Read the model definition and answer for the solid it produces. Units are mm, in the model's axes. Coordinates: 2 decimals unless noted, no trailing zeros. Order: outer loops, then holes, each group sorted by start corner. A loop starts at its lowest first (then second) coordinate and runs counter-clockwise, first axis right, second up. Notation, with made-up numbers: (1.5, 56.5) -> (22.5, 56.5) arc R6 ccw to (22.5, 65.5) -> close; hole circle Ø2 at (19, 4). An arc over 180 degrees is marked (long way). Answer as a JSON object with one key per item and string values. Group by question number.
1) Consider L1, parallel to Y at x = -84, z = 1.65; L2, parallel to Y at x = -152, z = 4.25; L3, parallel to X at y = 238, z = 2.35. Determine where each line is inside the solid, lowest interval first.
2) Section B-B on x = -83 is taken. Determine the outline of the cut face in (y, z).
3) Section A-A on y = 238.5 is taken. Determine the outline of the cut face in (x, z), and give its area (3 significant figures).
4) Section C-C on y = 31 is taken. Determine the outline of the cut face in (x, z).
5) Given pin 1 (1.5 mm diameter, centred on x = -56.5, z = 1.5, fed in from -Y); pin 2 (3 mm diameter, centred on x = -52, z = 2, fed in from +Y), each flat-ended and moving along its own axis, determine where each tip first touches the part or whether it passes through.
6) Section D-D on z = 3.7 is taken. Count the separate pieces of the cut face and the enclosed holes in it, and give its area (3 significant figures).
from build123d import *

# Parameters (mm, degrees)
BASE_DEPTH                = 5
ESQUISSE3_R               = 2
ESQUISSE3_W               = 65
ESQUISSE3_H               = 30
ENL_V_MAT_EXTRU_1_DEPTH   = 6
CONG_1_R                  = 3
PER_AGE_POUR_BILLES_REACH = 7
ESQUISSE6_R               = 2
ESQUISSE6_R_2             = 11
PER_AGE_POUR_PROFIL_REACH = 7
ESQUISSE8_R               = 3
ESQUISSE10_R              = 2
ENL_V_MAT_EXTRU_3_DEPTH   = 6
ESQUISSE13_R              = 2
ENL_V_MAT_EXTRU_4_DEPTH   = 10


with BuildPart() as part:
    # Esquisse1 → Base (new body)
    with BuildSketch(Plane.XY):
        Polygon((0, 0), (-175, 0), (-199.748737342, 24.748737342), (-199.748737342, 284.748737342), (-175, 309.497474683), (0, 309.497474683), (24.748737342, 284.748737342), (24.748737342, 24.748737342), align=None)
    extrude(amount=BASE_DEPTH)

    # Esquisse3 → Enlèv. mat.-Extru.1 (cut, through all)
    with BuildSketch(Plane(origin=(0, 0, 0), x_dir=(-1, 0, 0), z_dir=(0, 0, -1))):
        with Locations((52.5, 45)):
            Circle(ESQUISSE3_R)
        with Locations((122.5, 45)):
            Circle(ESQUISSE3_R)
        with Locations((122.5, 264.497474683)):
            Circle(ESQUISSE3_R)
        with Locations((52.5, 264.497474683)):
            Circle(ESQUISSE3_R)
        Polygon((129.5, 0), (129.5, 20), (105.5, 20), (105.5, 45.5), (69.5, 45.5), (69.5, 20), (45.5, 20), (45.5, 0), align=None)
        Polygon((45.5, 309.497474683), (129.5, 309.497474683), (129.5, 289.497474683), (105.5, 289.497474683), (105.5, 263.997474683), (69.5, 263.997474683), (69.5, 289.497474683), (45.5, 289.497474683), align=None)
        with Locations((87.5, 239.497474683)):
            Rectangle(ESQUISSE3_W, ESQUISSE3_H)
        with Locations((87.5, 70)):
            Rectangle(ESQUISSE3_W, ESQUISSE3_H)
    extrude(amount=-ENL_V_MAT_EXTRU_1_DEPTH, mode=Mode.SUBTRACT)

    # Congé1
    cong_1_edges = [part.edges().sort_by_distance(p)[0] for p in [
        (0, 0, 2.5),
        (-175, 0, 2.5),
        (-199.748737342, 24.748737342, 2.5),
        (-199.748737342, 284.748737342, 2.5),
        (-175, 309.497474683, 2.5),
        (0, 309.497474683, 2.5),
        (24.748737342, 284.748737342, 2.5),
        (24.748737342, 24.748737342, 2.5),
        (-45.5, 289.497474683, 2.5),
        (-45.5, 309.497474683, 2.5),
        (-129.5, 309.497474683, 2.5),
        (-129.5, 289.497474683, 2.5),
        (-105.5, 289.497474683, 2.5),
        (-105.5, 263.997474683, 2.5),
        (-69.5, 263.997474683, 2.5),
        (-69.5, 289.497474683, 2.5),
        (-129.5, 0, 2.5),
        (-45.5, 0, 2.5),
        (-45.5, 20, 2.5),
        (-69.5, 20, 2.5),
        (-69.5, 45.5, 2.5),
        (-105.5, 45.5, 2.5),
        (-105.5, 20, 2.5),
        (-129.5, 20, 2.5),
    ]]
    fillet(cong_1_edges, radius=CONG_1_R)

    # Esquisse6 → Perçage pour billes (cut, up to next)
    with BuildSketch(Plane.XY.offset(5), mode=Mode.PRIVATE) as per_age_pour_billes_sk1:
        with Locations((-1.784271247, 16)):
            Circle(ESQUISSE6_R)
    per_age_pour_billes_tool1 = extrude(per_age_pour_billes_sk1.sketch, amount=-PER_AGE_POUR_BILLES_REACH, mode=Mode.PRIVATE) & part.part
    add(per_age_pour_billes_tool1.solids().sort_by_distance((-1.784271, 16, 5))[0], mode=Mode.SUBTRACT)
    # Esquisse6 → Perçage pour billes (cut, up to next)
    with BuildSketch(Plane.XY.offset(5), mode=Mode.PRIVATE) as per_age_pour_billes_sk2:
        with Locations((-1.784271247, 46)):
            Circle(ESQUISSE6_R)
    per_age_pour_billes_tool2 = extrude(per_age_pour_billes_sk2.sketch, amount=-PER_AGE_POUR_BILLES_REACH, mode=Mode.PRIVATE) & part.part
    add(per_age_pour_billes_tool2.solids().sort_by_distance((-1.784271, 46, 5))[0], mode=Mode.SUBTRACT)
    # Esquisse6 → Perçage pour billes (cut, up to next)
    with BuildSketch(Plane.XY.offset(5), mode=Mode.PRIVATE) as per_age_pour_billes_sk3:
        with Locations((-1.784271247, 263.497474683)):
            Circle(ESQUISSE6_R)
    per_age_pour_billes_tool3 = extrude(per_age_pour_billes_sk3.sketch, amount=-PER_AGE_POUR_BILLES_REACH, mode=Mode.PRIVATE) & part.part
    add(per_age_pour_billes_tool3.solids().sort_by_distance((-1.784271, 263.497475, 5))[0], mode=Mode.SUBTRACT)
    # Esquisse6 → Perçage pour billes (cut, up to next)
    with BuildSketch(Plane.XY.offset(5), mode=Mode.PRIVATE) as per_age_pour_billes_sk4:
        with Locations((-1.784271247, 293.497474683)):
            Circle(ESQUISSE6_R)
    per_age_pour_billes_tool4 = extrude(per_age_pour_billes_sk4.sketch, amount=-PER_AGE_POUR_BILLES_REACH, mode=Mode.PRIVATE) & part.part
    add(per_age_pour_billes_tool4.solids().sort_by_distance((-1.784271, 293.497475, 5))[0], mode=Mode.SUBTRACT)
    # Esquisse6 → Perçage pour billes (cut, up to next)
    with BuildSketch(Plane.XY.offset(5), mode=Mode.PRIVATE) as per_age_pour_billes_sk5:
        with Locations((-1.784271247, 278.497474683)):
            Circle(ESQUISSE6_R_2)
    per_age_pour_billes_tool5 = extrude(per_age_pour_billes_sk5.sketch, amount=-PER_AGE_POUR_BILLES_REACH, mode=Mode.PRIVATE) & part.part
    add(per_age_pour_billes_tool5.solids().sort_by_distance((-1.784271, 278.497475, 5))[0], mode=Mode.SUBTRACT)
    # Esquisse6 → Perçage pour billes (cut, up to next)
    with BuildSketch(Plane.XY.offset(5), mode=Mode.PRIVATE) as per_age_pour_billes_sk6:
        with Locations((-1.784271247, 31)):
            Circle(ESQUISSE6_R_2)
    per_age_pour_billes_tool6 = extrude(per_age_pour_billes_sk6.sketch, amount=-PER_AGE_POUR_BILLES_REACH, mode=Mode.PRIVATE) & part.part
    add(per_age_pour_billes_tool6.solids().sort_by_distance((-1.784271, 31, 5))[0], mode=Mode.SUBTRACT)
    # Esquisse6 → Perçage pour billes (cut, up to next)
    with BuildSketch(Plane.XY.offset(5), mode=Mode.PRIVATE) as per_age_pour_billes_sk7:
        with Locations((-173.215728753, 16)):
            Circle(ESQUISSE6_R)
    per_age_pour_billes_tool7 = extrude(per_age_pour_billes_sk7.sketch, amount=-PER_AGE_POUR_BILLES_REACH, mode=Mode.PRIVATE) & part.part
    add(per_age_pour_billes_tool7.solids().sort_by_distance((-173.215729, 16, 5))[0], mode=Mode.SUBTRACT)
    # Esquisse6 → Perçage pour billes (cut, up to next)
    with BuildSketch(Plane.XY.offset(5), mode=Mode.PRIVATE) as per_age_pour_billes_sk8:
        with Locations((-173.215728753, 46)):
            Circle(ESQUISSE6_R)
    per_age_pour_billes_tool8 = extrude(per_age_pour_billes_sk8.sketch, amount=-PER_AGE_POUR_BILLES_REACH, mode=Mode.PRIVATE) & part.part
    add(per_age_pour_billes_tool8.solids().sort_by_distance((-173.215729, 46, 5))[0], mode=Mode.SUBTRACT)
    # Esquisse6 → Perçage pour billes (cut, up to next)
    with BuildSketch(Plane.XY.offset(5), mode=Mode.PRIVATE) as per_age_pour_billes_sk9:
        with Locations((-173.215728753, 31)):
            Circle(ESQUISSE6_R_2)
    per_age_pour_billes_tool9 = extrude(per_age_pour_billes_sk9.sketch, amount=-PER_AGE_POUR_BILLES_REACH, mode=Mode.PRIVATE) & part.part
    add(per_age_pour_billes_tool9.solids().sort_by_distance((-173.215729, 31, 5))[0], mode=Mode.SUBTRACT)
    # Esquisse6 → Perçage pour billes (cut, up to next)
    with BuildSketch(Plane.XY.offset(5), mode=Mode.PRIVATE) as per_age_pour_billes_sk10:
        with Locations((-173.215728753, 263.497474683)):
            Circle(ESQUISSE6_R)
    per_age_pour_billes_tool10 = extrude(per_age_pour_billes_sk10.sketch, amount=-PER_AGE_POUR_BILLES_REACH, mode=Mode.PRIVATE) & part.part
    add(per_age_pour_billes_tool10.solids().sort_by_distance((-173.215729, 263.497475, 5))[0], mode=Mode.SUBTRACT)
    # Esquisse6 → Perçage pour billes (cut, up to next)
    with BuildSketch(Plane.XY.offset(5), mode=Mode.PRIVATE) as per_age_pour_billes_sk11:
        with Locations((-173.215728753, 293.497474683)):
            Circle(ESQUISSE6_R)
    per_age_pour_billes_tool11 = extrude(per_age_pour_billes_sk11.sketch, amount=-PER_AGE_POUR_BILLES_REACH, mode=Mode.PRIVATE) & part.part
    add(per_age_pour_billes_tool11.solids().sort_by_distance((-173.215729, 293.497475, 5))[0], mode=Mode.SUBTRACT)
    # Esquisse6 → Perçage pour billes (cut, up to next)
    with BuildSketch(Plane.XY.offset(5), mode=Mode.PRIVATE) as per_age_pour_billes_sk12:
        with Locations((-173.215728753, 278.497474683)):
            Circle(ESQUISSE6_R_2)
    per_age_pour_billes_tool12 = extrude(per_age_pour_billes_sk12.sketch, amount=-PER_AGE_POUR_BILLES_REACH, mode=Mode.PRIVATE) & part.part
    add(per_age_pour_billes_tool12.solids().sort_by_distance((-173.215729, 278.497475, 5))[0], mode=Mode.SUBTRACT)

    # Esquisse8 → Perçage pour profilé (cut, up to next)
    with BuildSketch(Plane.XY.offset(5), mode=Mode.PRIVATE) as per_age_pour_profil_sk1:
        with Locations((-152.5, 23)):
            Circle(ESQUISSE8_R)
    per_age_pour_profil_tool1 = extrude(per_age_pour_profil_sk1.sketch, amount=-PER_AGE_POUR_PROFIL_REACH, mode=Mode.PRIVATE) & part.part
    add(per_age_pour_profil_tool1.solids().sort_by_distance((-152.5, 23, 5))[0], mode=Mode.SUBTRACT)
    # Esquisse8 → Perçage pour profilé (cut, up to next)
    with BuildSketch(Plane.XY.offset(5), mode=Mode.PRIVATE) as per_age_pour_profil_sk2:
        with Locations((-152.5, 286.497474683)):
            Circle(ESQUISSE8_R)
    per_age_pour_profil_tool2 = extrude(per_age_pour_profil_sk2.sketch, amount=-PER_AGE_POUR_PROFIL_REACH, mode=Mode.PRIVATE) & part.part
    add(per_age_pour_profil_tool2.solids().sort_by_distance((-152.5, 286.497475, 5))[0], mode=Mode.SUBTRACT)
    # Esquisse8 → Perçage pour profilé (cut, up to next)
    with BuildSketch(Plane.XY.offset(5), mode=Mode.PRIVATE) as per_age_pour_profil_sk3:
        with Locations((-22.5, 286.497474683)):
            Circle(ESQUISSE8_R)
    per_age_pour_profil_tool3 = extrude(per_age_pour_profil_sk3.sketch, amount=-PER_AGE_POUR_PROFIL_REACH, mode=Mode.PRIVATE) & part.part
    add(per_age_pour_profil_tool3.solids().sort_by_distance((-22.5, 286.497475, 5))[0], mode=Mode.SUBTRACT)
    # Esquisse8 → Perçage pour profilé (cut, up to next)
    with BuildSketch(Plane.XY.offset(5), mode=Mode.PRIVATE) as per_age_pour_profil_sk4:
        with Locations((-22.5, 23)):
            Circle(ESQUISSE8_R)
    per_age_pour_profil_tool4 = extrude(per_age_pour_profil_sk4.sketch, amount=-PER_AGE_POUR_PROFIL_REACH, mode=Mode.PRIVATE) & part.part
    add(per_age_pour_profil_tool4.solids().sort_by_distance((-22.5, 23, 5))[0], mode=Mode.SUBTRACT)

    # Esquisse10 → Enlèv. mat.-Extru.3 (cut, through all)
    with BuildSketch(Plane.XY.offset(5)):
        with Locations((-120.5, 214.497474683)):
            Circle(ESQUISSE10_R)
        with Locations((-120.5, 166.197474683)):
            Circle(ESQUISSE10_R)
        with Locations((-54.5, 166.197474683)):
            Circle(ESQUISSE10_R)
        with Locations((-54.5, 214.497474683)):
            Circle(ESQUISSE10_R)
        with Locations((-54.5, 143.3)):
            Circle(ESQUISSE10_R)
        with Locations((-54.5, 95)):
            Circle(ESQUISSE10_R)
        with Locations((-120.5, 143.3)):
            Circle(ESQUISSE10_R)
        with Locations((-120.5, 95)):
            Circle(ESQUISSE10_R)
    extrude(amount=-ENL_V_MAT_EXTRU_3_DEPTH, mode=Mode.SUBTRACT)

    # Esquisse13 → Enlèv. mat.-Extru.4 (cut)
    with BuildSketch(Plane.XY.offset(5)):
        with Locations((-20.251262658, 204.748737342)):
            Circle(ESQUISSE13_R)
        with Locations((-20.251262658, 184.748737342)):
            Circle(ESQUISSE13_R)
        with Locations((-20.251262658, 124.748737342)):
            Circle(ESQUISSE13_R)
        with Locations((-20.251262658, 104.748737342)):
            Circle(ESQUISSE13_R)
    extrude(amount=-ENL_V_MAT_EXTRU_4_DEPTH, mode=Mode.SUBTRACT)


solid = part.part
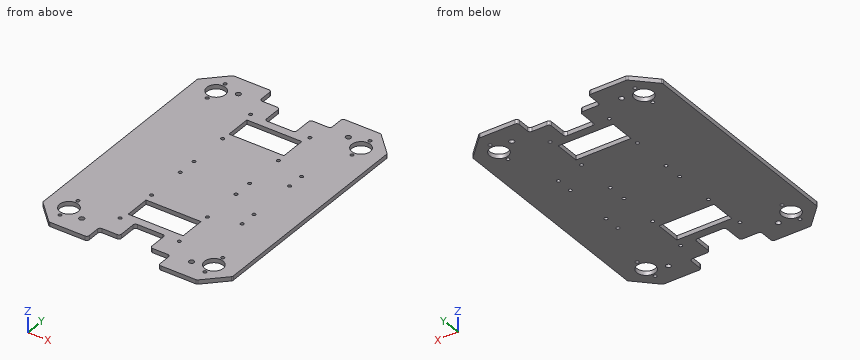
Worked answers:
{
 "1": {"L1": "y = 45.5 to 55, 85 to 224.5, 254.5 to 264", "L2": "y = 0 to 20.04, 25.96 to 283.54, 289.46 to 309.5", "L3": "x = -199.75 to -120, -55 to 24.75"},
 "2": {"outline": "(45.5, 0) -> (55, 0) -> (55, 5) -> (45.5, 5) -> close; (85, 0) -> (224.5, 0) -> (224.5, 5) -> (85, 5) -> close; (254.5, 0) -> (264, 0) -> (264, 5) -> (254.5, 5) -> close"},
 "3": {"outline": "(-199.75, 0) -> (-120, 0) -> (-120, 5) -> (-199.75, 5) -> close; (-55, 0) -> (24.75, 0) -> (24.75, 5) -> (-55, 5) -> close", "area": "797 mm²"},
 "4": {"outline": "(-199.75, 0) -> (-184.22, 0) -> (-184.22, 5) -> (-199.75, 5) -> close; (-162.22, 0) -> (-105.5, 0) -> (-105.5, 5) -> (-162.22, 5) -> close; (-69.5, 0) -> (-12.78, 0) -> (-12.78, 5) -> (-69.5, 5) -> close; (9.22, 0) -> (24.75, 0) -> (24.75, 5) -> (9.22, 5) -> close"},
 "5": {"pin 1": "stops at y = 20", "pin 2": "stops at y = 289.5"},
 "6": {"separate pieces": "1", "enclosed holes": "34", "area": "57,200 mm²"}
}
